```python
from build123d import *

# Parameters (mm, degrees)
F0_W      = 29.15
F0_H      = 59.5
F0_W_2    = 24.15
F0_H_2    = 54.5
F1_DEPTH  = 2
F2_DEPTH  = 15
F3_W      = 2
F3_H      = 13
F4_DEPTH  = 25
F6_DEPTH  = 15
F5_W      = 24.15
F5_H      = 7.5
F7_DEPTH  = 2
F8_R      = 2.1
F9_DEPTH  = 5
F10_R     = 1.6
F11_DEPTH = 25


with BuildPart() as f1:
    # F0 (on Top) → F1 (new body)
    with BuildSketch(Plane.XY):
        Rectangle(F0_W, F0_H)
        Rectangle(F0_W_2, F0_H_2, mode=Mode.SUBTRACT)
        Rectangle(F0_W_2, F0_H_2)
    extrude(amount=F1_DEPTH)

    # F0 (on Top) → F2 (join)
    with BuildSketch(Plane.XY):
        Rectangle(F0_W, F0_H)
        Rectangle(F0_W_2, F0_H_2, mode=Mode.SUBTRACT)
    extrude(amount=F2_DEPTH)

    # F3 (on face) → F4 (cut)
    with BuildSketch(Plane(origin=(0, -27.25, 0), x_dir=(-1, 0, 0), z_dir=(0, 1, 0))):
        with Locations((11.075, 8.5)):
            Rectangle(F3_W, F3_H)
        with Locations((-11.075, 8.5)):
            Rectangle(F3_W, F3_H)
    extrude(amount=-F4_DEPTH, mode=Mode.SUBTRACT)

    # F5 (on face) → F6 (join)
    with BuildSketch(Plane(origin=(0, 0, 0), x_dir=(1, 0, 0), z_dir=(0, 0, -1))):
        Polygon((-14.575, 39.75), (-14.575, 29.75), (-12.075, 29.75), (-12.075, 37.25), (12.075, 37.25), (12.075, 29.75), (14.575, 29.75), (14.575, 39.75), align=None)
    extrude(amount=-F6_DEPTH)

    # F5 (on face) → F7 (join)
    with BuildSketch(Plane(origin=(0, 0, 0), x_dir=(1, 0, 0), z_dir=(0, 0, -1))):
        with Locations((0, 33.5)):
            Rectangle(F5_W, F5_H)
    extrude(amount=-F7_DEPTH)

    # F8 (on face) → F9 (cut)
    with BuildSketch(Plane.XZ.offset(39.75)):
        with Locations((0, 7.5)):
            Circle(F8_R)
    extrude(amount=-F9_DEPTH, mode=Mode.SUBTRACT)

    # F10 (on face) → F11 (cut)
    with BuildSketch(Plane(origin=(0, 29.75, 0), x_dir=(-1, 0, 0), z_dir=(0, 1, 0))):
        with Locations((0, 7.5)):
            Circle(F10_R)
    extrude(amount=-F11_DEPTH, mode=Mode.SUBTRACT)


solid = f1.part
```
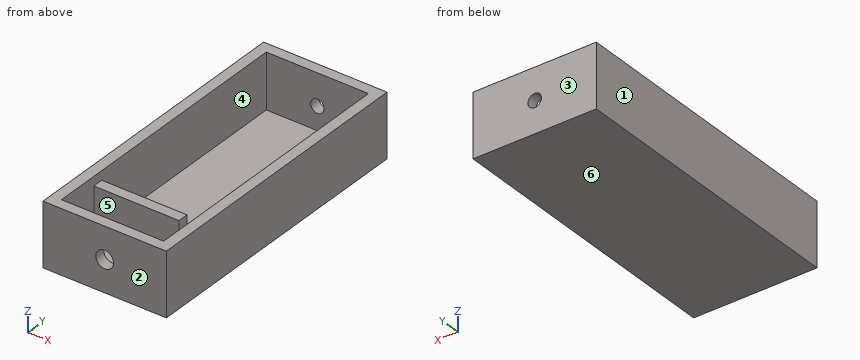
Could you check a few things on this model? Use its own coordinates, in mm. Face numbers are marked on the shaded views. A direction names the side the tool comes from. Give positions to 0.01 mm unless a question says otherwise; leave off trailing zeros. Write each loop counter-clockwise with the first axis right and the second up, starting at its lowest first coordinate (ties: lowest second). Pieces come first, ordered by that corner, then holes. Notation, with made-up numbers: (-15, 39.25) - (20, 39.25) arc R15 ccw to (20, 59.25) - close; hole circle Ø7 at (17.25, 28). An arc over 180 degrees is marked (long way). One line per item, written item: value. Start each with the question number.
Item 1: Imagine slicing it at D-D, the plane y = -17. List the corners of the cut face in (x, z) for me (3 decimals), and give its area (3 significant figures).
Item 2: If we mould it in two halves opening along Y, with no side actions, what happens to the marked faces 1, 2, 3 and 4? For each: +Y half, -Y half, draft (parallel to the pull), parting line (faces both ways), or undercut.
Item 3: I'm going to push a flat-ended pin straight in: pin 1 (2 mm diameter, centred on x = 2, y = -19.5, fed in from +Z). Where does the tip first touch, or does it pass through?
Item 4: Imagine slicing it at B-B, the plane x = 0. List the corners of the cut face in (y, z) for me.
Item 5: Which directions (+Z, -Z, +X, -X, +Y, -Y) give clear straight access to the entire face, cutting with the end or side of a thin tool? Please do the marked faces 5 and 6.
Item 6: Imagine slicing it at A-A, the plane z = 12.75. List the corners of the cut face in (x, y) for me (3 decimals).
Item 7: Imagine slicing it at C-C, the plane z = 7.5. List the corners of the cut face in (x, y) for me (3 decimals).
Item 8: Please list where these lines run through material, in increasing order: line 1 (Y direction, x = -3.25, z = 12); line 2 (X direction, y = -29, z = 13.25) (3 decimals); line 3 (Z direction, x = 0, y = -37.9). Write a range as from..to.
Geometry says:
1. outline: (-14.575, 0) - (14.575, 0) - (14.575, 15) - (12.075, 15) - (12.075, 2) - (-12.075, 2) - (-12.075, 15) - (-14.575, 15) - close
1. area: 123 mm^2
2. face 1: draft
2. face 2: -Y half
2. face 3: +Y half
2. face 4: undercut
3. pin 1: z = 2
4. outline: (-39.75, 0) - (29.75, 0) - (29.75, 5.9) - (27.25, 5.9) - (27.25, 2) - (-27.25, 2) - (-27.25, 15) - (-29.75, 15) - (-29.75, 2) - (-37.25, 2) - (-37.25, 5.4) - (-39.75, 5.4) - close; (-39.75, 9.6) - (-37.25, 9.6) - (-37.25, 15) - (-39.75, 15) - close; (27.25, 9.1) - (29.75, 9.1) - (29.75, 15) - (27.25, 15) - close
5. face 5: +Z
5. face 6: -Z, +X, -X, +Y, -Y
6. outline: (-14.575, -39.75) - (14.575, -39.75) - (14.575, 29.75) - (-14.575, 29.75) - close; (-10.075, -29.75) - (10.075, -29.75) - (10.075, -27.25) - (-10.075, -27.25) - close; hole (-12.075, -37.25) - (12.075, -37.25) - (12.075, 27.25) - (-12.075, 27.25) - close
7. outline: (-14.575, -39.75) - (-2.1, -39.75) - (-2.1, -37.25) - (-12.075, -37.25) - (-12.075, 27.25) - (-1.6, 27.25) - (-1.6, 29.75) - (-14.575, 29.75) - close; (-10.075, -29.75) - (10.075, -29.75) - (10.075, -27.25) - (-10.075, -27.25) - close; (1.6, 27.25) - (12.075, 27.25) - (12.075, -37.25) - (2.1, -37.25) - (2.1, -39.75) - (14.575, -39.75) - (14.575, 29.75) - (1.6, 29.75) - close
8. line 1: -39.75..-37.25, -29.75..-27.25, 27.25..29.75
8. line 2: -14.575..-12.075, -10.075..10.075, 12.075..14.575
8. line 3: 0..5.4, 9.6..15
